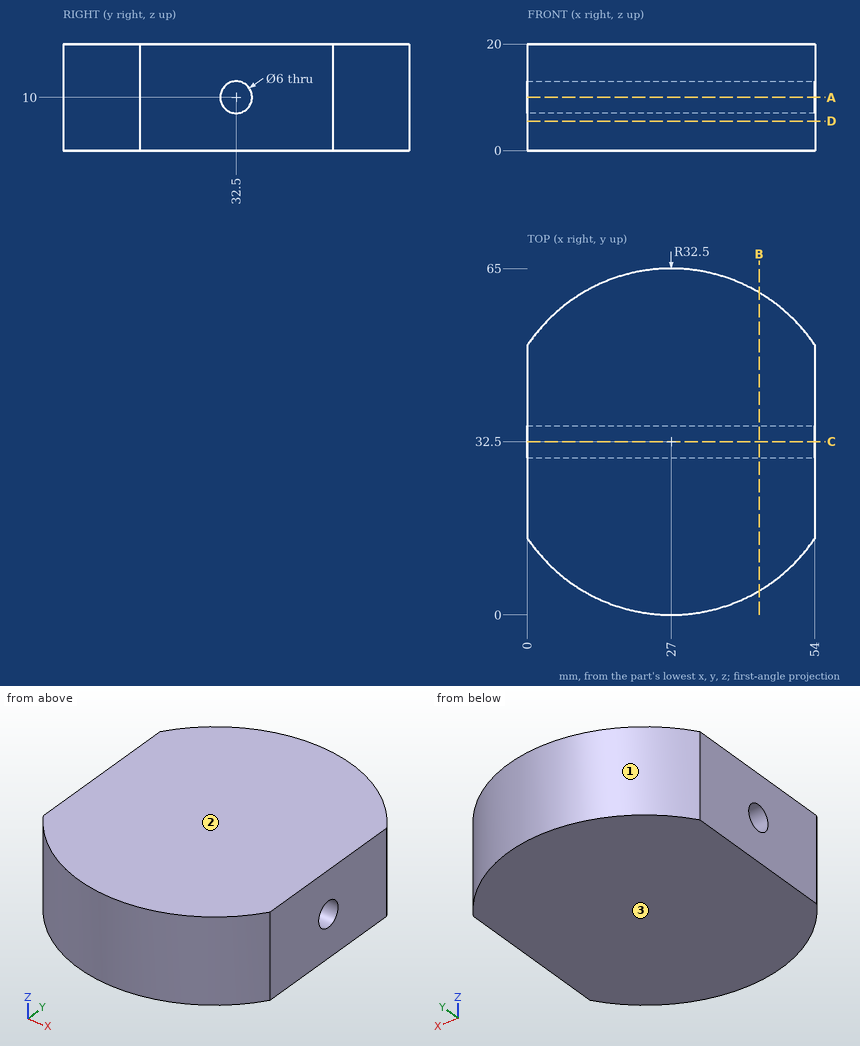
Answer from the drawing. Dimensions are ordinates in mm from the lowest x, y and z of the part. Coordinates: 2 decimals unless noted, no trailing zeros. Write each loop counter-clockwise with the first axis right and the second up, starting at its lowest first coordinate (ties: lowest second). Pieces come first, ordered by that corner, then holes. Notation, with made-up numbers: M -16.75,16 L 19.25,16 A18 ccw 19.25,31 Z; hole C 2.5,87.5 d6. An arc over 180 degrees is marked long. Write item = value, one per line.
1. Straight lines are drawn through the part: line 1 (Y direction, x = 28.5, z = 9.25); line 2 (Y direction, x = 7.5, z = 10); line 3 (Z direction, x = 20, y = 32). For each, find the intervals that lie inside material, in ascending order. Write a range as from..to.
Solution:
line_1 = 0.03..29.6, 35.4..64.97
line_2 = 6.5..29.5, 35.5..58.5
line_3 = 0..7.04, 12.96..20
2. The part is cut by section D-D (z = 5.5). Determine the outline of the cut face in (x, y).
Solution:
outline = M 0,14.41 A32.5 ccw 54,14.41 L 54,50.59 A32.5 ccw 0,50.59 Z
3. The part is cut by section B-B (x = 43.5). Determine the outline of the cut face in (y, z).
Solution:
outline = M 4.5,0 L 60.5,0 L 60.5,20 L 4.5,20 Z; hole C 32.5,10 d6
4. The part is cut by section C-C (y = 32.5). Determine the outline of the cut face in (x, z).
Solution:
outline = M 0,0 L 54,0 L 54,7 L 0,7 Z; M 0,13 L 54,13 L 54,20 L 0,20 Z
5. The part is cut by section A-A (z = 10). Determine the outline of the cut face in (x, y).
Solution:
outline = M 0,14.41 A32.5 ccw 54,14.41 L 54,29.5 L 0,29.5 Z; M 0,35.5 L 54,35.5 L 54,50.59 A32.5 ccw 0,50.59 Z
6. Flat-ended cylindrical pins translate along their axes: pin 1 (4 mm diameter, centred on x = 12.5, z = 13.5, fed in from +Y); pin 2 (8 mm diameter, centred on x = 38, z = 16, fed in from -Y); pin 3 (4 mm diameter, centred on x = 40.5, z = 2, fed in from +Y). Find the tip coordinate at first contact, or state that the pin passes through.
Solution:
pin_1 = 62.5
pin_2 = 0.76
pin_3 = 62.9
7. Determine the mould class of the marked faces 1, 2 and 3 for opening direction Z: released by +Z, released by -Z, zero draft, split by the parting line, or undercut.
Solution:
face_1 = zero draft
face_2 = released by +Z
face_3 = released by -Z
